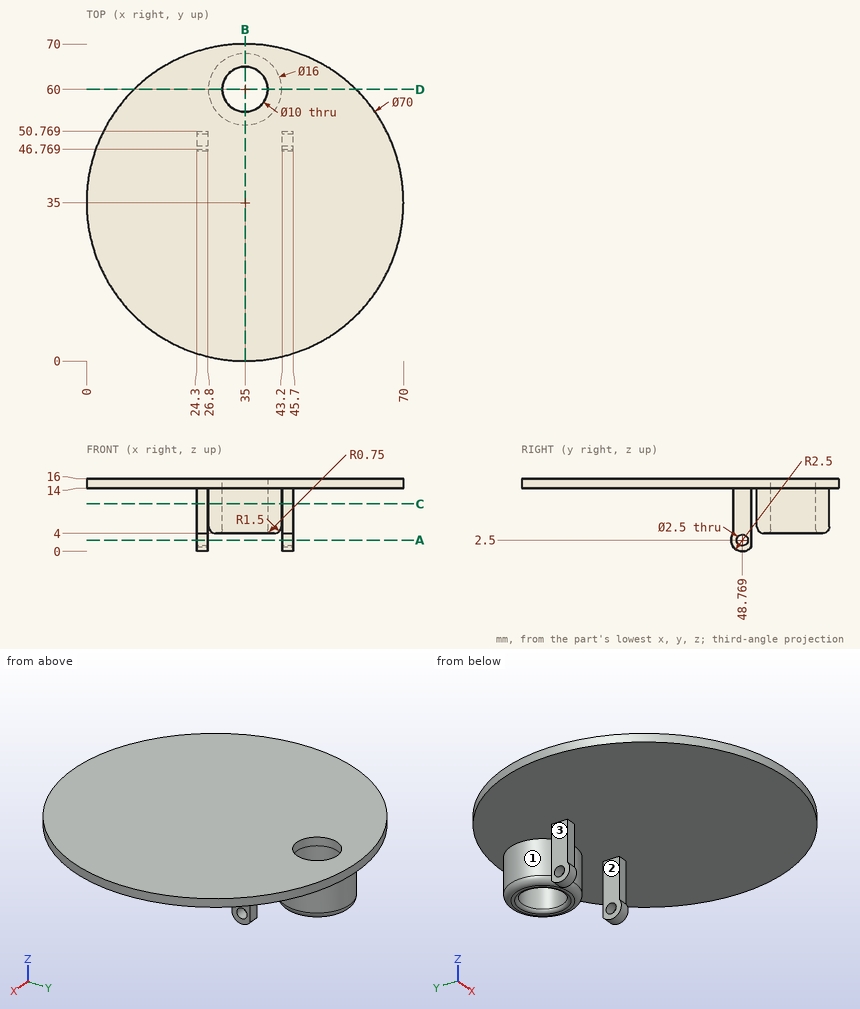
The drawing under review shows one solid part. Ordinate dimensions are in mm from its lowest x, y, z. Round coordinates to 2 decimals unless told otherwise and drop trailing zeros. Order: outer loops, then holes, each group sorted by start corner. A loop starts at its lowest first (then second) coordinate and runs counter-clockwise, first axis right, second up. Notation, with made-up numbers: (-1, 70) -> (5, 70) arc R12 ccw to (5, 82) -> close; hole circle Ø2 at (25.5, 50.25). An arc over 180 degrees is marked (long way). Use a Markdown table: item, result.
Q1. We need section D-D on y = 60. Write out the cut boundary in (x, z) (3 decimals), then the cut area to 3 significant figures.
Values:
| item | result |
|---|---|
| outline | (10.505, 14) -> (27, 14) -> (27, 5.5) arc R1.5 ccw to (28.5, 4) -> (29.25, 4) arc R0.75 ccw to (30, 4.75) -> (30, 16) -> (10.505, 16) -> close; (40, 4.75) arc R0.75 ccw to (40.75, 4) -> (41.5, 4) arc R1.5 ccw to (43, 5.5) -> (43, 14) -> (59.495, 14) -> (59.495, 16) -> (40, 16) -> close |
| area | 137 mm^2 |
Q2. Clearance check with flat-ended pins moving along their axes: P1, Ø1.2, axis at x = 44, z = 7, coming from the +Y side; P2, Ø2, axis at y = 49, z = 9, coming from the -X side; P3, Ø3, axis at x = 45, z = 6.5, coming from the -Y side; P4, Ø2, axis at y = 48.77, z = 2.5, coming from the +X side. State where each tip first meets the part, or that it passes through.
Values:
| item | result |
|---|---|
| P1 | stops at y = 50.77 |
| P2 | stops at x = 24.3 |
| P3 | stops at y = 46.77 |
| P4 | passes through |
Q3. Mouldability with a two-part tool opening along X and no side actions: class the marked faces 1, 2 and 3 as +X half, -X half, draft (parallel to the pull), parting line (faces both ways), or undercut.
Values:
| item | result |
|---|---|
| face 1 | parting line |
| face 2 | undercut |
| face 3 | -X half |
Q4. For line 1 (Y direction, x = 35, z = 12.25); line 2 (X direction, y = 60, z = 9); line 3 (X direction, y = 50.5, z = 5), list the stretches that pass through material, from the lowest coordinate up.
Values:
| item | result |
|---|---|
| line 1 | y = 52 to 55, 65 to 68 |
| line 2 | x = 27 to 30, 40 to 43 |
| line 3 | x = 24.3 to 26.8, 43.2 to 45.7 |
Q5. We need section B-B on x = 35. Write out the cut boundary in (y, z), then the cut area to 3 significant figures.
Values:
| item | result |
|---|---|
| outline | (0, 14) -> (52, 14) -> (52, 5.5) arc R1.5 ccw to (53.5, 4) -> (54.25, 4) arc R0.75 ccw to (55, 4.75) -> (55, 16) -> (0, 16) -> close; (65, 4.75) arc R0.75 ccw to (65.75, 4) -> (66.5, 4) arc R1.5 ccw to (68, 5.5) -> (68, 14) -> (70, 14) -> (70, 16) -> (65, 16) -> close |
| area | 179 mm^2 |
Q6. We need section C-C on z = 10.5. Write out the cut boundary in (x, y).
Values:
| item | result |
|---|---|
| outline | (24.3, 46.77) -> (26.8, 46.77) -> (26.8, 50.77) -> (24.3, 50.77) -> close; circle Ø16 at (35, 60); (43.2, 46.77) -> (45.7, 46.77) -> (45.7, 50.77) -> (43.2, 50.77) -> close; hole circle Ø10 at (35, 60) |
Q7. We need section A-A on z = 2.5. Write out the cut boundary in (x, y), then the cut area to 3 significant figures.
Values:
| item | result |
|---|---|
| outline | (24.3, 46.27) -> (26.8, 46.27) -> (26.8, 47.52) -> (24.3, 47.52) -> close; (24.3, 50.02) -> (26.8, 50.02) -> (26.8, 50.77) -> (24.3, 50.77) -> close; (43.2, 46.27) -> (45.7, 46.27) -> (45.7, 47.52) -> (43.2, 47.52) -> close; (43.2, 50.02) -> (45.7, 50.02) -> (45.7, 50.77) -> (43.2, 50.77) -> close |
| area | 10.0 mm^2 |
